Build history of the part. All positions in model axes, mm. A direction names the side the tool comes from. Give positions to 0.01 mm unless a question says otherwise; leave off trailing zeros. Order: outer loops, then holes, each group sorted by start corner. A loop starts at its lowest first (then second) coordinate and runs counter-clockwise, first axis right, second up. Notation, with made-up numbers: (69, 7) -> (114, 7) arc R5 ccw to (114, 14) -> close; hole circle Ø4 at (-40, 47.25). An arc over 180 degrees is marked (long way). One line per item, written item: value. Start each with the question number.
(1) Probe line 1 (Z direction, x = -1.5, y = -113); line 2 (X direction, y = -26.5, z = -1); line 3 (X direction, y = -157.5, z = 13). List the from-to ranges inside material, lowest first.
(2) Pin check, flat tips, straight feed: pin 1 (4 mm diameter, centred on x = -38, y = -126.5, fed in from +Z); pin 2 (6 mm diameter, centred on x = -23, y = -89.5, fed in from -Z); pin 3 (4 mm diameter, centred on y = -139.5, z = 21, fed in from +X); pin 4 (6 mm diameter, centred on x = 8.5, z = 44, fed in from +Y). Stop position of each tip, or through.
(3) Which spindle directions (+Z, -Z, +X, -X, +Y, -Y) get a long thin tool onto all of the face, cutting with end or side? Do faces 4 (the cylindrical face through (-41.777, -168.384, 0.519)), 5 (the flat face through (-1, -81, 31.964)), 6 (the flat face through (49, -169.912, 1)). Say none if no direction does.
(4) Saw through at B-B on x = 0. Give the cut face in (y, z).
(5) Two-plate mould, pull along Z, no slides. Class faces 1 (the cylindrical face through (-16.267, -83.767, -73.256)), 2 (the flat face through (-1.1, 0, -32.3)), 3 (the cylindrical face through (0.64, -168.38, 33.41)): +Z half, -Z half, draft (parallel to the pull), parting line (faces both ways), or undercut.
(6) Saw through at A-A on z = 0. Give the cut face in (x, y), plus the area to 3 significant figures.
(7) Saw through at D-D on z = -43.5. Give the cut face in (x, y).
(8) Saw through at C-C on y = -145.5. Give the cut face in (x, z), plus the area to 3 significant figures.
```python
from build123d import *

# Parameters (mm, degrees)
F0_R     = 75.040734
F0_W     = 80.655844
F0_H     = 63.927502
F1_DEPTH = 169.911919
F2_R     = 5.08
F3_SIZE  = 5.08


with BuildPart() as f1:
    # F0 (on Front) → F1 (new body)
    with BuildSketch(Plane.XZ):
        Circle(F0_R)
        Rectangle(F0_W, F0_H, mode=Mode.SUBTRACT)
    extrude(amount=F1_DEPTH)

    # F2
    f2_edges = [f1.edges().sort_by_distance(p)[0] for p in [
        (0, -169.911919, 31.963751),
        (-40.327922, -169.911919, 0),
    ]]
    fillet(f2_edges, radius=F2_R)

    # F3
    f3_edges = [f1.edges().sort_by_distance(p)[0] for p in [
        (40.327922, -169.911919, 0),
        (0, -169.911919, -31.963751),
    ]]
    chamfer(f3_edges, length=F3_SIZE)


solid = f1.part
```
Results below:
1. line 1: z = -75.03 to -31.96, 31.96 to 75.03
1. line 2: x = -75.03 to -40.33, 40.33 to 75.03
1. line 3: x = -73.91 to -40.33, 40.33 to 73.91
2. pin 1: stops at z = 65.84
2. pin 2: stops at z = -72.33
2. pin 3: stops at x = 72.6
2. pin 4: stops at y = 0
3. face 4: -Y
3. face 5: +Y, -Y
3. face 6: +Z, -Z, +X, -X, -Y
4. outline: (-169.91, -75.04) -> (0, -75.04) -> (0, -31.96) -> (-164.83, -31.96) -> (-169.91, -37.04) -> close; (-169.91, 37.04) arc R5.08 ccw to (-164.83, 31.96) -> (0, 31.96) -> (0, 75.04) -> (-169.91, 75.04) -> close
5. face 1: parting line
5. face 2: draft
5. face 3: undercut
6. outline: (-75.04, -169.91) -> (-45.41, -169.91) arc R5.08 ccw to (-40.33, -164.83) -> (-40.33, 0) -> (-75.04, 0) -> close; (40.33, -164.83) -> (45.41, -169.91) -> (75.04, -169.91) -> (75.04, 0) -> (40.33, 0) -> close
6. area: 11,800 mm²
7. outline: (-61.15, -169.91) -> (61.15, -169.91) -> (61.15, 0) -> (-61.15, 0) -> close
8. outline: circle Ø150.08 at (0, 0); hole (-40.33, -31.96) -> (40.33, -31.96) -> (40.33, 31.96) -> (-40.33, 31.96) -> close
8. area: 12,500 mm²
